Study the drawing (mm; zero at the part's minimum x, y, z) and answer. A direction names the side the tool comes from. Coordinates: 2 decimals unless noted, no trailing zeros. Order: outer loops, then holes, each group sorted by start corner. A loop starts at its lowest first (then second) coordinate and runs counter-clockwise, first axis right, second up.
1. The part is cut by section C-C, the plane x = 447. Give the vertices of the cut face in (y, z), then the cut area to 3 significant figures.
2. Flat-ended cylindrical pins translate along their axes: pin 1 Ø1.5 at (y, z) = (575, 207.5) entering from -X; pin 2 Ø1 at (x, y) = (423, 238.5) entering from +Z; pin 3 Ø6 at (y, z) = (122.5, 232) entering from -X. Find the tip coordinate at first contact, or state that the pin passes through.
3. Determine the mould class of the marked faces 4, 5, 6 and 7 for opening direction Y: +Y half, -Y half, draft (parallel to the pull), parting line (faces both ways), or undercut.
4. The part is cut by section A-A, the plane z = 184. Give the vertices of the cut face in (x, y).
5. Find the intervals of material crossed by probe 1 along Y at (x, z) = (162, 30.5); probe 2 along X at (y, z) = (27, 279); probe 3 along X at (y, z) = (305.5, 106), in increasing order.
6. A tool of negligible diameter and unlimited length cuts with its end or side. For the marked faces 1, 2 and 3, from which of +Z, -Z, +X, -X, +Y, -Y can it reach the whole face along a straight path? Write none if from no direction.
7. The part is cut by section B-B, the plane y = 174.5. Give the vertices of the cut face in (x, z), then the cut area to 3 significant figures.
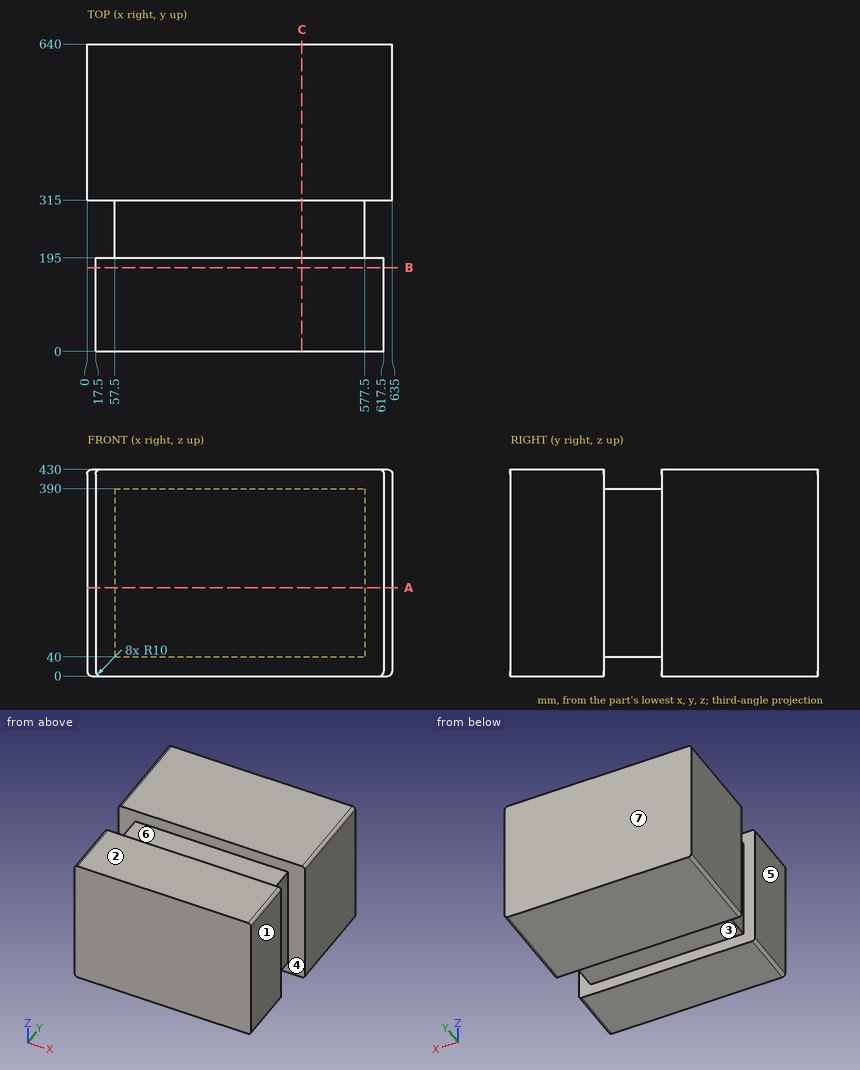
Geometry says:
1. outline: (0, 0) - (195, 0) - (195, 40) - (315, 40) - (315, 0) - (640, 0) - (640, 430) - (315, 430) - (315, 390) - (195, 390) - (195, 430) - (0, 430) - close
1. area: 266,000 mm2
2. pin 1: stops at x = 0
2. pin 2: stops at z = 390
2. pin 3: stops at x = 17.5
3. face 4: undercut
3. face 5: draft
3. face 6: undercut
3. face 7: +Y half
4. outline: (0, 315) - (57.5, 315) - (57.5, 195) - (17.5, 195) - (17.5, 0) - (617.5, 0) - (617.5, 195) - (577.5, 195) - (577.5, 315) - (635, 315) - (635, 640) - (0, 640) - close
5. probe 1: y = 0 to 195, 315 to 640
5. probe 2: x = 17.5 to 617.5
5. probe 3: x = 57.5 to 577.5
6. face 1: +Z, -Z, +X, -Y
6. face 2: +Z, +X, -X, +Y, -Y
6. face 3: -Z, +X, -X
7. outline: (17.5, 10) arc R10 ccw to (27.5, 0) - (607.5, 0) arc R10 ccw to (617.5, 10) - (617.5, 420) arc R10 ccw to (607.5, 430) - (27.5, 430) arc R10 ccw to (17.5, 420) - close
7. area: 258,000 mm2
